```python
from build123d import *

# Parameters (mm, degrees)
SKETCH1_R                   = 9.525
SKETCH1_R_2                 = 8.5471
BOSS_EXTRUDE1_DEPTH         = 31
F_41_0_096_DIAMETER_HOLE1_D = 2.4384
CHAMFER1_SIZE               = 0.5


with BuildPart() as part:
    # Sketch1 → Boss-Extrude1 (new, symmetric)
    with BuildSketch(Plane(origin=(0, 0, 0), x_dir=(1, 0, 0), z_dir=(0, 1, 0))):
        with Locations(Location((0, 0, 0), (0, 0, 270))):
            Circle(SKETCH1_R)
        with Locations(Location((0, 0, 0), (0, 0, 270))):
            Circle(SKETCH1_R_2, mode=Mode.SUBTRACT)
    extrude(amount=BOSS_EXTRUDE1_DEPTH, both=True)

    # 41 _0.096_ Diameter Hole1 (through all)
    with Locations(Plane.ZY.offset(9.525)):
        with Locations((0, 28), (0, -28)):
            Hole(F_41_0_096_DIAMETER_HOLE1_D / 2)

    # Chamfer1
    chamfer1_edges = [part.edges().sort_by_distance(p)[0] for p in [
        (0, 31, -9.525),
        (0, -31, -9.525),
    ]]
    chamfer(chamfer1_edges, length=CHAMFER1_SIZE)


solid = part.part
```
For this review, take the finished solid that the model builds, in its own axes (mm). Coordinates: 2 decimals unless noted, no trailing zeros. Write each loop counter-clockwise with the first axis right and the second up, starting at its lowest first coordinate (ties: lowest second). Pieces come first, ordered by that corner, then holes.
(1) Add section A-A on z = 0. Give the boundary of the cut face in (x, y) (3 decimals), then the cut area to 3 significant figures.
(2) Add section B-B on x = 0. Give the boundary of the cut face in (y, z) (3 decimals), then the cut area to 3 significant figures.
(3) For pin 1 Ø6 at (x, y) = (3.5, -23) entering from -Z, flat-tipped, find the tip position at first contact; note if it passes through.
(4) Add section C-C on y = -28. Give the boundary of the cut face in (x, z) (3 decimals).
(5) Wall thickness on probe 1 along Y at (x, z) = (9, 0); probe 2 along X at (y, z) = (-16.5, 0) (3 decimals); probe 3 along Y at (x, z) = (9.35, 0) (3 decimals): over which ranges is each line inside the solid? List them lowest first.
Answer sheet:
1. outline: (-9.525, -30.5) - (-9.025, -31) - (-8.547, -31) - (-8.547, -29.219) - (-9.525, -29.219) - close; (-9.525, -26.781) - (-8.547, -26.781) - (-8.547, 26.781) - (-9.525, 26.781) - close; (-9.525, 29.219) - (-8.547, 29.219) - (-8.547, 31) - (-9.025, 31) - (-9.525, 30.5) - close; (8.547, -31) - (9.025, -31) - (9.525, -30.5) - (9.525, -29.219) - (8.547, -29.219) - close; (8.547, -26.781) - (9.525, -26.781) - (9.525, 26.781) - (8.547, 26.781) - close; (8.547, 29.219) - (9.525, 29.219) - (9.525, 30.5) - (9.025, 31) - (8.547, 31) - close
1. area: 111 mm2
2. outline: (-31, -9.025) - (-30.5, -9.525) - (30.5, -9.525) - (31, -9.025) - (31, -8.547) - (-31, -8.547) - close; (-31, 8.547) - (31, 8.547) - (31, 9.025) - (30.5, 9.525) - (-30.5, 9.525) - (-31, 9.025) - close
2. area: 121 mm2
3. pin 1: stops at z = -9.51
4. outline: (-9.447, -1.219) arc R9.525 ccw to (9.447, -1.219) - (8.46, -1.219) arc R8.547 cw to (-8.46, -1.219) - close; (-9.447, 1.219) - (-8.46, 1.219) arc R8.547 cw to (8.46, 1.219) - (9.447, 1.219) arc R9.525 ccw to start
5. probe 1: y = -31 to -29.22, -26.78 to 26.78, 29.22 to 31
5. probe 2: x = -9.525 to -8.547, 8.547 to 9.525
5. probe 3: y = -30.675 to -29.219, -26.781 to 26.781, 29.219 to 30.675
